Geometry: final body of the model. Coordinates: model frame, mm. A direction names the side the tool comes from. Round coordinates to 2 decimals unless told otherwise and drop trailing zeros. Loops run counter-clockwise (first coordinate to the right, second up) from the corner with the lowest first, then second, coordinate; pieces in that order, holes last. Notation, with made-up numbers: (3.25, 10) -> (50.25, 10) arc R18 ccw to (50.25, 22) -> close; hole circle Ø1 at (-26.75, -23). An arc over 180 degrees is marked (long way). Answer in a Markdown table with one row per item.
```python
from build123d import *

# Parameters (mm, degrees)
F0_R      = 190
F1_DEPTH  = 55
F2_R      = 45
F3_DEPTH  = 20
F4_R      = 176
F4_R_2    = 136
F5_DEPTH  = 5
F5_FACE_R = 136
F6_DEPTH  = 15


with BuildPart() as f1:
    # F0 (on Front) → F1 (new body)
    with BuildSketch(Plane.XZ):
        Circle(F0_R)
    extrude(amount=F1_DEPTH)

    # F2 (on face) → F3 (cut)
    with BuildSketch(Plane(origin=(0, 0, 0), x_dir=(-1, 0, 0), z_dir=(0, 1, 0))):
        Circle(F2_R)
    extrude(amount=-F3_DEPTH, mode=Mode.SUBTRACT)

    # F4 (on face) → F5 (cut)
    with BuildSketch(Plane.XZ.offset(55)):
        Circle(F4_R)
        Circle(F4_R_2, mode=Mode.SUBTRACT)
    extrude(amount=-F5_DEPTH, mode=Mode.SUBTRACT)

    # F5_face (on face) → F6 (cut)
    with BuildSketch(Plane.XZ.offset(55)):
        Circle(F5_FACE_R)
    extrude(amount=-F6_DEPTH, mode=Mode.SUBTRACT)


solid = f1.part
```
Item 1: Cut plane B-B (x = 0). Output: boundary loops of the cut face in (y, z).
Answer:
| item | result |
|---|---|
| outline | (-55, -190) -> (0, -190) -> (0, -45) -> (-20, -45) -> (-20, 45) -> (0, 45) -> (0, 190) -> (-55, 190) -> (-55, 176) -> (-50, 176) -> (-50, 136) -> (-40, 136) -> (-40, -136) -> (-50, -136) -> (-50, -176) -> (-55, -176) -> close |
Item 2: Cut plane D-D (z = -127.5). Output: boundary loops of the cut face in (x, y), then the cut area to 3 significant figures.
Answer:
| item | result |
|---|---|
| outline | (-140.87, -55) -> (-121.32, -55) -> (-121.32, -50) -> (-47.33, -50) -> (-47.33, -40) -> (47.33, -40) -> (47.33, -50) -> (121.32, -50) -> (121.32, -55) -> (140.87, -55) -> (140.87, 0) -> (-140.87, 0) -> close |
| area | 13,300 mm² |
Item 3: Pin query (flat end, axial travel): pin 1 Ø12 at (x, z) = (-36.5, -123) entering from -Y; pin 2 Ø5 at (y, z) = (-20, 21.5) entering from +X; pin 3 Ø12 at (y, z) = (-20, -72) entering from -X. Return the tip coordinate at first contact, or that it passes through.
Answer:
| item | result |
|---|---|
| pin 1 | stops at y = -40 |
| pin 2 | stops at x = 189.05 |
| pin 3 | stops at x = -178.17 |
Item 4: Cut plane A-A (z = 0). Output: boundary loops of the cut face in (x, y), then the cut area to 3 significant figures.
Answer:
| item | result |
|---|---|
| outline | (-190, -55) -> (-176, -55) -> (-176, -50) -> (-136, -50) -> (-136, -40) -> (136, -40) -> (136, -50) -> (176, -50) -> (176, -55) -> (190, -55) -> (190, 0) -> (45, 0) -> (45, -20) -> (-45, -20) -> (-45, 0) -> (-190, 0) -> close |
| area | 14,600 mm² |
Item 5: Draft query along Z for faces 1 (the face through (-20.765, -9.86, -39.923)), 2 (the face through (168, -55, -55)), 3 (the face through (-38.153, -52.535, -171.815)), 4 (the face through (-41.19, -27.12, -185.48)). Return one class per face: pulls with the +Z half, pulls with the -Z half, needs draft (parallel to the pull), parting line crosses it, or undercut.
Answer:
| item | result |
|---|---|
| face 1 | undercut |
| face 2 | needs draft |
| face 3 | undercut |
| face 4 | parting line crosses it |
Item 6: Cut plane C-C (y = -29.5). Output: boundary loops of the cut face in (x, z), then the cut area to 3 significant figures.
Answer:
| item | result |
|---|---|
| outline | circle Ø380 at (0, 0) |
| area | 113,000 mm² |
Item 7: Line query: probe 1 along Z at (x, y) = (0, -46); probe 2 along Z at (x, y) = (0, -53.1); probe 3 along Y at (x, z) = (136, -78.5). Output: solid intervals per line, ascending. Write a range as [from, to].
Answer:
| item | result |
|---|---|
| probe 1 | z = [-190, -136], [136, 190] |
| probe 2 | z = [-190, -176], [176, 190] |
| probe 3 | y = [-50, 0] |
Item 8: Reachability of faces 5 (the face through (90, -50, -103)), 6 (the face through (1, -20, 1)), 7 (the face through (40, 0, -40)) from +Z, -Z, +X, -X, +Y, -Y: full face, straight path, thin tool, end or side. Return the list, or none.
Answer:
| item | result |
|---|---|
| face 5 | -Y |
| face 6 | +Y |
| face 7 | +Z, -Z, +X, -X, +Y |
